```python
from build123d import *

# Parameters (mm, degrees)
SKETCH1_R                                        = 571.5
SKETCH1_W                                        = 736.6
SKETCH1_H                                        = 736.6
BOSS_EXTRUDE1_DEPTH                              = 9.525
SKETCH3_R                                        = 3.96875
CUT_EXTRUDE1_DEPTH                               = 809.279175548
F_3_8_CLEARANCE_HOLE1_D                          = 10.31748
CIRPATTERN_16X_3_8_CLEARANCE_HOLES_COUNT         = 16
F_1_4_BOX_HOLES_2_D                              = 6.7564
LPATTERN1_COUNT                                  = 6
LPATTERN1_PITCH                                  = 127
LPATTERN1_COUNT_DIR2                             = 2
LPATTERN1_PITCH_DIR2                             = 800.1
F_1_4_BOX_HOLES_1_D                              = 6.7564
LPATTERN2_COUNT                                  = 6
LPATTERN2_PITCH                                  = 127
LPATTERN2_COUNT_DIR2                             = 2
LPATTERN2_PITCH_DIR2                             = 800.1
CSK_FOR_1_4_FLAT_HEAD_MACHINE_SCREW1_D           = 6.7564
CSK_FOR_1_4_FLAT_HEAD_MACHINE_SCREW1_CSINK_D     = 12.8778
CSK_FOR_1_4_FLAT_HEAD_MACHINE_SCREW1_CSINK_ANGLE = 82
CIRPATTERN4_COUNT                                = 8
FILLET1_R                                        = 6.35


with BuildPart() as part:
    # Sketch1 → Boss-Extrude1 (new body)
    with BuildSketch(Plane(origin=(0, 0, 0), x_dir=(1, 0, 0), z_dir=(0, 1, 0))):
        with Locations(Location((0, 0, 0), (0, 0, 90))):
            Circle(SKETCH1_R)
        Rectangle(SKETCH1_W, SKETCH1_H, mode=Mode.SUBTRACT)
    extrude(amount=BOSS_EXTRUDE1_DEPTH)

    # Sketch3 → Cut-Extrude1 (cut, through all)
    with BuildSketch(Plane(origin=(0, 9.525, 0), x_dir=(1, 0, 0), z_dir=(0, 1, 0))):
        with Locations(Location((-554.0375, 0, 0), (0, 0, 270))):
            Circle(SKETCH3_R)
        with BuildLine():
            Line((547.6875, 3.96875), (560.3875, 3.96875))
            ThreePointArc((560.3875, 3.96875), (564.35625, 0), (560.3875, -3.96875))
            Line((560.3875, -3.96875), (547.6875, -3.96875))
            ThreePointArc((547.6875, -3.96875), (543.71875, 0), (547.6875, 3.96875))
        make_face()
    extrude(amount=-CUT_EXTRUDE1_DEPTH, mode=Mode.SUBTRACT)

    # 3/8 Clearance Hole1 (through all)
    with Locations(Plane(origin=(0, 0, 0), x_dir=(-1, 0, 0), z_dir=(0, -1, 0))):
        with Locations((-543.391824791, -108.087354284)):
            f_3_8_clearance_hole1 = Hole(F_3_8_CLEARANCE_HOLE1_D / 2)

    # CirPattern - 16X 3/8 Clearance Holes: 3/8 Clearance Hole1 ×16 about axis
    cirpattern_16x_3_8_clearance_holes_axis = Axis((0, 0, 0), (0, 1, 0))
    for i in range(1, CIRPATTERN_16X_3_8_CLEARANCE_HOLES_COUNT):
        add(f_3_8_clearance_hole1.rotate(cirpattern_16x_3_8_clearance_holes_axis, i * 360 / CIRPATTERN_16X_3_8_CLEARANCE_HOLES_COUNT), mode=Mode.SUBTRACT)

    # 1/4 Box Holes 2 (through all)
    with Locations(Plane(origin=(0, 9.525, 0), x_dir=(1, 0, 0), z_dir=(0, 1, 0))):
        with Locations((-317.5, -400.05)):
            f_1_4_box_holes_2 = Hole(F_1_4_BOX_HOLES_2_D / 2)

    # LPattern1: 1_4 Box Holes 2 6 × 2
    with Locations(*[(i * LPATTERN1_PITCH, 0, -j * LPATTERN1_PITCH_DIR2) for i in range(LPATTERN1_COUNT) for j in range(LPATTERN1_COUNT_DIR2) if (i, j) != (0, 0)]):
        add(f_1_4_box_holes_2, mode=Mode.SUBTRACT)

    # 1/4 Box Holes 1 (through all)
    with Locations(Plane(origin=(0, 9.525, 0), x_dir=(1, 0, 0), z_dir=(0, 1, 0))):
        with Locations((-400.05, -317.5)):
            f_1_4_box_holes_1 = Hole(F_1_4_BOX_HOLES_1_D / 2)

    # LPattern2: 1_4 Box Holes 1 6 × 2
    with Locations(*[(j * LPATTERN2_PITCH_DIR2, 0, -i * LPATTERN2_PITCH) for i in range(LPATTERN2_COUNT) for j in range(LPATTERN2_COUNT_DIR2) if (i, j) != (0, 0)]):
        add(f_1_4_box_holes_1, mode=Mode.SUBTRACT)

    # CSK for 1/4 Flat Head Machine Screw1 (through all)
    with Locations(Plane(origin=(0, 0, 0), x_dir=(-1, 0, 0), z_dir=(0, -1, 0))):
        with Locations((-511.863906494, 212.020972159)):
            csk_for_1_4_flat_head_machine_screw1 = CounterSinkHole(CSK_FOR_1_4_FLAT_HEAD_MACHINE_SCREW1_D / 2, CSK_FOR_1_4_FLAT_HEAD_MACHINE_SCREW1_CSINK_D / 2, counter_sink_angle=CSK_FOR_1_4_FLAT_HEAD_MACHINE_SCREW1_CSINK_ANGLE)

    # CirPattern4: CSK for 1/4 Flat Head Machine Screw1 ×8 about axis
    cirpattern4_axis = Axis((0, 0, 0), (0, 1, 0))
    for i in range(1, CIRPATTERN4_COUNT):
        add(csk_for_1_4_flat_head_machine_screw1.rotate(cirpattern4_axis, i * 360 / CIRPATTERN4_COUNT), mode=Mode.SUBTRACT)

    # Fillet1
    fillet1_edges = [part.edges().sort_by_distance(p)[0] for p in [
        (-368.3, 4.7625, -368.3),
        (-368.3, 4.7625, 368.3),
        (368.3, 4.7625, 368.3),
        (368.3, 4.7625, -368.3),
    ]]
    fillet(fillet1_edges, radius=FILLET1_R)


solid = part.part
```
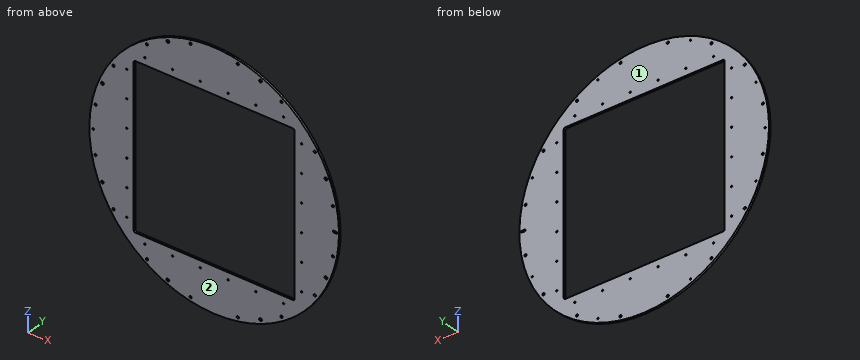
Check sheet for the modelled part. Datum: model origin and axes. Units: mm. Face numbers are marked on the shaded views. Coordinates: 2 decimals unless noted, no trailing zeros. Write each loop counter-clockwise with the first axis right and the second up, starting at its lowest first coordinate (ties: lowest second). Pieces come first, ordered by that corner, then holes. Notation, with made-up numbers: M -9.5,40.25 L 48.5,40.25 A31 ccw 48.5,70.25 Z; hole C -30.75,-1 d1. An arc over 180 degrees is marked long. Write item = value, one per line. Start each with the question number.
1. Thickness scan on probe 1 along X at (y, z) = (6.5, 192); probe 2 along Z at (x, y) = (190.5, 4); probe 3 along Z at (x, y) = (12.5, 7.5). Record the ranges inside material, lowest first.
2. Mould release check, pull along Y, two halves, no side actions. Record for the marked faces 1 and 2: pulls with the +Y half, pulls with the -Y half, needs draft (parallel to the pull), parting line crosses it, or undercut.
3. Sectioned sample at A-A (z = 35). Record the cut outline in (x, y) (3 decimals).
4. Go/stop test with flat-tipped pins: pin 1 (1 mm diameter, centred on y = 5, z = -280.5, fed in from +X); pin 2 (11 mm diameter, centred on x = -400.05, z = -63.5, fed in from -Y); pin 3 (5 mm diameter, centred on x = 387, y = 3.5, fed in from +Z); pin 4 (5 mm diameter, centred on y = 3.5, z = 165, fed in from -X). Record where each tip stops, or that it passes through.
5. Sectioned sample at C-C (z = 277.5). Record the cut outline in (x, y) (3 decimals), then the cut area to 3 significant figures.
6. Sectioned sample at B-B (y = 6.25). State how many separate pieces and enclosed holes the cut face has, then the cut area to 3 significant figures.
The answers:
q1.probe_1 = -538.28 to -403.08, -397.02 to -368.3, 368.3 to 397.02, 403.08 to 538.28
q1.probe_2 = -538.82 to -403.43, -396.67 to -368.3, 368.3 to 396.67, 403.43 to 538.82
q1.probe_3 = -571.36 to -368.3, 368.3 to 571.36
q2.face_1 = pulls with the +Y half
q2.face_2 = pulls with the -Y half
q3.outline = M -570.427,0 L -368.3,0 L -368.3,9.525 L -570.427,9.525 Z; M 368.3,0 L 570.427,0 L 570.427,9.525 L 368.3,9.525 Z
q4.pin_1 = 498.21
q4.pin_2 = 0
q4.pin_3 = 422.81
q4.pin_4 = -547.91
q5.outline = M -499.606,0 L -368.3,0 L -368.3,9.525 L -499.606,9.525 Z; M 368.3,0 L 499.606,0 L 499.606,9.525 L 368.3,9.525 Z
q5.area = 2,500 mm²
q6.separate_pieces = 1
q6.enclosed_holes = 51
q6.area = 481,000 mm²
